Geometry: final body of the model. Coordinates: model frame, mm. A direction names the side the tool comes from. Coordinates: 2 decimals unless noted, no trailing zeros. Loops run counter-clockwise (first coordinate to the right, second up) from the corner with the lowest first, then second, coordinate; pieces in that order, holes last. Notation, with made-up numbers: (67, 12.25) - (122, 12.25) arc R28 cw to (122, 42.25) - close; hole circle Ø11 at (73, 40). An arc over 180 degrees is marked (long way). Return JSON: item names as keys, results as strings.
from build123d import *

# Parameters (mm, degrees)
F1_DEPTH = 2
F2_DEPTH = 19
F3_R     = 2.75
F3_R_2   = 1.25
F4_DEPTH = 5
F5_W     = 9
F5_H     = 0.5
F5_W_2   = 17
F5_W_3   = 8
F5_W_4   = 0.5
F5_H_2   = 15.1
F5_H_3   = 15.9
F6_DEPTH = 12
F7_W     = 15.6
F7_H     = 4
F8_DEPTH = 0.5


with BuildPart() as f1:
    # F0 (on Top) → F1 (new body)
    with BuildSketch(Plane.XY):
        with BuildLine():
            Line((88.5, 62.5), (2.5, 62.5))
            ThreePointArc((2.5, 62.5), (0.3786796564, 61.6213203436), (-0.5, 59.5))
            Line((-0.5, 59.5), (-0.5, 2.5))
            ThreePointArc((-0.5, 2.5), (0.3786796564, 0.3786796564), (2.5, -0.5))
            Line((2.5, -0.5), (88.5, -0.5))
            ThreePointArc((88.5, -0.5), (90.6213203436, 0.3786796564), (91.5, 2.5))
            Line((91.5, 2.5), (91.5, 59.5))
            ThreePointArc((91.5, 59.5), (90.6213203436, 61.6213203436), (88.5, 62.5))
        make_face()
        with BuildLine():
            Line((88.5, 0), (2.5, 0))
            ThreePointArc((2.5, 0), (0.732233047, 0.732233047), (0, 2.5))
            Line((0, 2.5), (0, 59.5))
            ThreePointArc((0, 59.5), (0.732233047, 61.267766953), (2.5, 62))
            Line((2.5, 62), (88.5, 62))
            ThreePointArc((88.5, 62), (90.267766953, 61.267766953), (91, 59.5))
            Line((91, 59.5), (91, 2.5))
            ThreePointArc((91, 2.5), (90.267766953, 0.732233047), (88.5, 0))
        make_face(mode=Mode.SUBTRACT)
        with BuildLine():
            ThreePointArc((0, 2.5), (0.732233047, 0.732233047), (2.5, 0))
            Line((2.5, 0), (88.5, 0))
            ThreePointArc((88.5, 0), (90.267766953, 0.732233047), (91, 2.5))
            Line((91, 2.5), (91, 59.5))
            ThreePointArc((91, 59.5), (90.267766953, 61.267766953), (88.5, 62))
            Line((88.5, 62), (2.5, 62))
            ThreePointArc((2.5, 62), (0.732233047, 61.267766953), (0, 59.5))
            Line((0, 59.5), (0, 2.5))
        make_face()
    extrude(amount=F1_DEPTH)

    # F0 (on Top) → F2 (join)
    with BuildSketch(Plane.XY):
        with BuildLine():
            Line((88.5, 62.5), (2.5, 62.5))
            ThreePointArc((2.5, 62.5), (0.3786796564, 61.6213203436), (-0.5, 59.5))
            Line((-0.5, 59.5), (-0.5, 2.5))
            ThreePointArc((-0.5, 2.5), (0.3786796564, 0.3786796564), (2.5, -0.5))
            Line((2.5, -0.5), (88.5, -0.5))
            ThreePointArc((88.5, -0.5), (90.6213203436, 0.3786796564), (91.5, 2.5))
            Line((91.5, 2.5), (91.5, 59.5))
            ThreePointArc((91.5, 59.5), (90.6213203436, 61.6213203436), (88.5, 62.5))
        make_face()
        with BuildLine():
            Line((88.5, 0), (2.5, 0))
            ThreePointArc((2.5, 0), (0.732233047, 0.732233047), (0, 2.5))
            Line((0, 2.5), (0, 59.5))
            ThreePointArc((0, 59.5), (0.732233047, 61.267766953), (2.5, 62))
            Line((2.5, 62), (88.5, 62))
            ThreePointArc((88.5, 62), (90.267766953, 61.267766953), (91, 59.5))
            Line((91, 59.5), (91, 2.5))
            ThreePointArc((91, 2.5), (90.267766953, 0.732233047), (88.5, 0))
        make_face(mode=Mode.SUBTRACT)
    extrude(amount=F2_DEPTH)

    # F3 (on face) → F4 (join)
    with BuildSketch(Plane.XY.offset(2)):
        with Locations((6.5, 55.5)):
            Circle(F3_R)
        with Locations((6.5, 55.5)):
            Circle(F3_R_2, mode=Mode.SUBTRACT)
        with Locations((64.5, 55.5)):
            Circle(F3_R)
        with Locations((64.5, 55.5)):
            Circle(F3_R_2, mode=Mode.SUBTRACT)
        with Locations((6.5, 6.5)):
            Circle(F3_R)
        with Locations((6.5, 6.5)):
            Circle(F3_R_2, mode=Mode.SUBTRACT)
        with Locations((64.5, 6.5)):
            Circle(F3_R)
        with Locations((64.5, 6.5)):
            Circle(F3_R_2, mode=Mode.SUBTRACT)
    extrude(amount=F4_DEPTH)

    # F5 (on face) → F6 (cut)
    with BuildSketch(Plane.XY.offset(19)):
        with Locations((13.05, -0.25)):
            Rectangle(F5_W, F5_H)
        with Locations((34.5, -0.25)):
            Rectangle(F5_W_2, F5_H)
        with Locations((56.75, -0.25)):
            Rectangle(F5_W_3, F5_H)
        with Locations((91.25, 50.45)):
            Rectangle(F5_W_4, F5_H_2)
        with Locations((91.25, 31.45)):
            Rectangle(F5_W_4, F5_H_2)
        with Locations((91.25, 12.75)):
            Rectangle(F5_W_4, F5_H_3)
    extrude(amount=-F6_DEPTH, mode=Mode.SUBTRACT)

    # F7 (on face) → F8 (cut)
    with BuildSketch(Plane(origin=(-0.5, 0, 0), x_dir=(0, -1, 0), z_dir=(-1, 0, 0))):
        with Locations((-32.2, 6)):
            Rectangle(F7_W, F7_H)
    extrude(amount=-F8_DEPTH, mode=Mode.SUBTRACT)


solid = f1.part
Item 1: Mould query, pull axis X, two halves, no side actions, for faces 3 (the face through (77.2, -0.2, 19)), 4 (the face through (91.5, 31, 5)), 5 (the face through (6, 7, 2)). Classes: +X half, -X half, draft (parallel to the pull), parting line (faces both ways), or undercut.
Worked out:
{"face 3": "draft", "face 4": "+X half", "face 5": "undercut"}
Item 2: Reachability of faces 1 (the face through (45, 31, 0)), 2 (the face through (6, 56, 2)) from +Z, -Z, +X, -X, +Y, -Y: full face, straight path, thin tool, end or side. Return the list, or none.
Worked out:
{"face 1": "-Z, +X, -X, +Y, -Y", "face 2": "+Z"}
Item 3: Section query A-A, the plane z = 5.75. Count the separate pieces of the cut face and the enclosed holes in it, and give its area (3 significant figures).
Worked out:
{"separate pieces": "5", "enclosed holes": "4", "area": "219 mm^2"}
Item 4: First-contact query: pin 1 Ø12 at (x, y) = (48, 17) entering from -Z; pin 2 Ø2 at (x, y) = (6.5, 55.5) entering from +Z; pin 3 Ø5 at (x, z) = (57.5, 10.5) entering from -Y; pin 4 Ø1.6 at (x, y) = (5.5, 7) entering from +Z. Flat tips, straight axial feed; report the tip coordinate or a pass-through.
Worked out:
{"pin 1": "z = 0", "pin 2": "z = 2", "pin 3": "y = 62", "pin 4": "z = 7"}
Item 5: Section query D-D, the plane y = 13.5. Return loops of the section in (x, z), and give its area (3 significant figures).
Worked out:
{"outline": "(-0.5, 0) - (91.5, 0) - (91.5, 7) - (91, 7) - (91, 2) - (0, 2) - (0, 19) - (-0.5, 19) - close", "area": "195 mm^2"}
Item 6: Section query C-C, the plane x = 6.5. Return loops of the section in (y, z).
Worked out:
{"outline": "(-0.5, 0) - (62.5, 0) - (62.5, 19) - (62, 19) - (62, 2) - (58.25, 2) - (58.25, 7) - (56.75, 7) - (56.75, 2) - (54.25, 2) - (54.25, 7) - (52.75, 7) - (52.75, 2) - (9.25, 2) - (9.25, 7) - (7.75, 7) - (7.75, 2) - (5.25, 2) - (5.25, 7) - (3.75, 7) - (3.75, 2) - (0, 2) - (0, 19) - (-0.5, 19) - close"}
Item 7: Ray query, probe 1 along Y at (x, z) = (6.5, 5.45); probe 2 along Y at (x, z) = (30, 2.5); probe 3 along X at (y, z) = (42, 2.25). Return the intervals inside material, ascending. Write a range as from..to.
Worked out:
{"probe 1": "-0.5..0, 3.75..5.25, 7.75..9.25, 52.75..54.25, 56.75..58.25, 62..62.5", "probe 2": "-0.5..0, 62..62.5", "probe 3": "-0.5..0, 91..91.5"}
Item 8: Section query B-B, the plane y = 37.5. Return loops of the section in (x, z), and give its area (3 significant figures).
Worked out:
{"outline": "(-0.5, 0) - (91.5, 0) - (91.5, 7) - (91, 7) - (91, 2) - (0, 2) - (0, 4) - (-0.5, 4) - close; (-0.5, 8) - (0, 8) - (0, 19) - (-0.5, 19) - close", "area": "193 mm^2"}
